Here's the drawing with two shaded views (mm, measured from the low corner). I have some questions. A direction names the side the tool comes from. Coordinates: 2 decimals unless noted, no trailing zeros. Order: outer loops, then holes, each group sorted by start corner. A loop starts at its lowest first (then second) coordinate and runs counter-clockwise, first axis right, second up. Notation, with made-up numbers: (-28, -9) -> (16, -9) arc R21 cw to (16, 18) -> close; hole circle Ø3 at (28.5, 61.25). An arc over 180 degrees is marked (long way). Answer in a Markdown table with one row per item. Add a question column.
1. If I drill on line 1 along X through (y, z) = (48, 38); line 2 along Y through (x, z) = (43, 9), over which ranges is the centre line in solid material (lowest first)? Write a range as [from, to].
2. Imagine slicing it at A-A on x = 25. Write out the boundary of the cut face in (y, z).
3. Imagine slicing it at C-C on y = 14. Write out the boundary of the cut face in (x, z).
4. On a 3-axis mill with a long thin cutter (end or side, diameter ignored), from which of +Z, -Z, +X, -X, +Y, -Y can I reach the whole of each face in a straight line? I mean the marked faces 5 and 6. Say none if no direction works.
5. Imagine slicing it at D-D on y = 25.4. State how many separate pieces and enclosed holes the cut face has, plus the area to 3 significant figures.
6. We'd pull the mould along Y, two halves only. Please class the marked faces 1, 2, 3 and 4: pulls with the +Y half, pulls with the -Y half, needs draft (parallel to the pull), parting line crosses it, or undercut.
7. Will these pins go through, and if not, where does the flat tip stop? pin 1 (5 mm diameter, centred on x = 17, y = 48.5, fed in from +Z); pin 2 (3.5 mm diameter, centred on y = 7.44, z = 4.9, fed in from +X); pin 3 (1.5 mm diameter, centred on x = 43.5, z = 7.5, fed in from -Y).
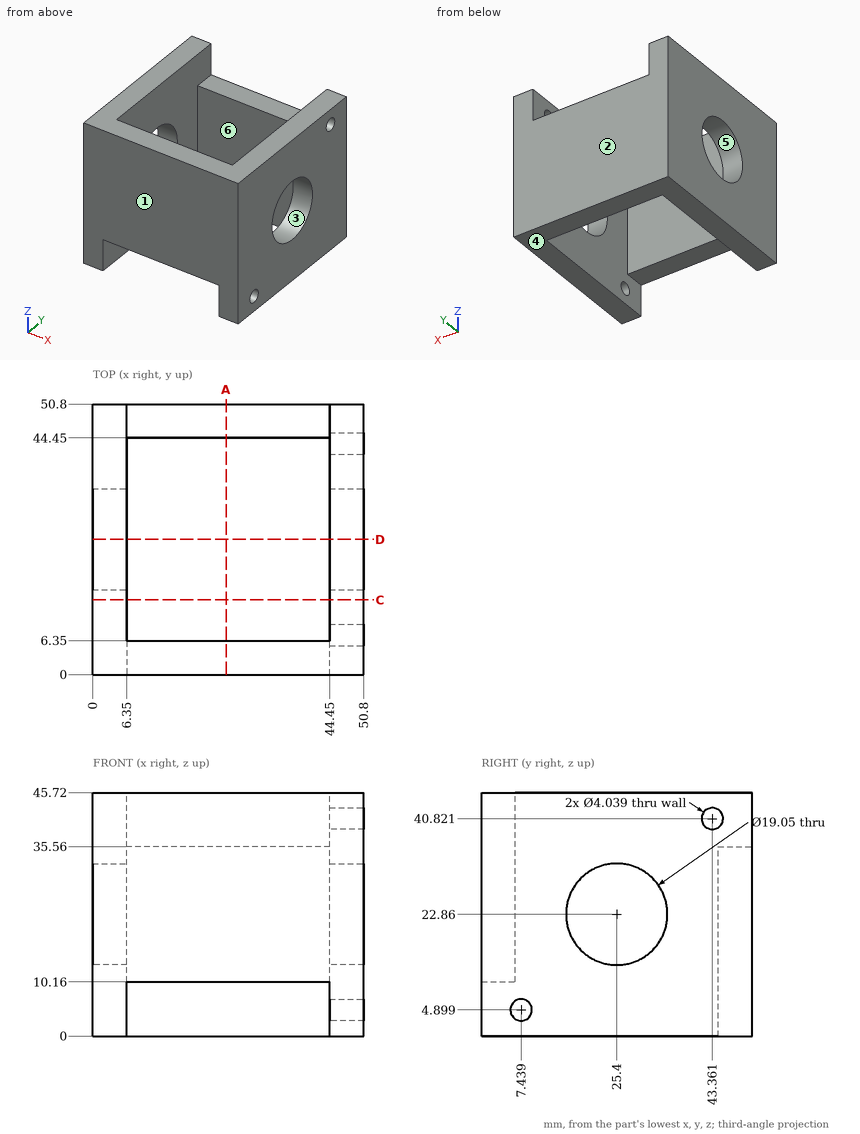
Answers follow:
| question | item | result |
|---|---|---|
| 1 | line 1 | x = [0, 6.35], [44.45, 50.8] |
| 1 | line 2 | y = [44.45, 50.8] |
| 2 | outline | (0, 10.16) -> (6.35, 10.16) -> (6.35, 45.72) -> (0, 45.72) -> close; (44.45, 0) -> (50.8, 0) -> (50.8, 35.56) -> (44.45, 35.56) -> close |
| 3 | outline | (0, 0) -> (6.35, 0) -> (6.35, 45.72) -> (0, 45.72) -> close; (44.45, 0) -> (50.8, 0) -> (50.8, 45.72) -> (44.45, 45.72) -> close |
| 4 | face 5 | +X, -X |
| 4 | face 6 | +Z, -Z |
| 5 | separate pieces | 4 |
| 5 | enclosed holes | 0 |
| 5 | area | 339 mm² |
| 6 | face 1 | pulls with the -Y half |
| 6 | face 2 | pulls with the +Y half |
| 6 | face 3 | undercut |
| 6 | face 4 | needs draft |
| 7 | pin 1 | stops at z = 35.56 |
| 7 | pin 2 | stops at x = 6.35 |
| 7 | pin 3 | stops at y = 44.45 |
